from build123d import *

# Parameters (mm, degrees)
BOSS_EXTRUDE1_DEPTH         = 2.75
FILLET1_R                   = 12.7
SKETCH5_R                   = 1.3890625
CUT_EXTRUDE4_DEPTH          = 3.75
CIRPATTERN2_COUNT           = 3
CIRPATTERN2_COPY_1_SKETCH_R = 1.3890625
CIRPATTERN2_COPY_1_DEPTH    = 3.75
CIRPATTERN2_COPY_2_SKETCH_R = 1.3890625
CIRPATTERN2_COPY_2_DEPTH    = 3.75


with BuildPart() as part:
    # Sketch1 → Boss-Extrude1 (new body)
    with BuildSketch(Plane(origin=(0, 0, 0), x_dir=(1, 0, 0), z_dir=(0, 1, 0))):
        Polygon((-22.265317244, 97.17689372), (22.265317244, 97.17689372), (95.290317244, -29.306116503), (73.025, -67.870777217), (-73.025, -67.870777217), (-95.290317244, -29.306116503), align=None)
    extrude(amount=BOSS_EXTRUDE1_DEPTH)

    # Fillet1
    fillet1_edges = [part.edges().sort_by_distance(p)[0] for p in [
        (-22.265317244, 1.375, -97.17689372),
        (22.265317244, 1.375, -97.17689372),
        (95.290317244, 1.375, 29.306116503),
        (73.025, 1.375, 67.870777217),
        (-73.025, 1.375, 67.870777217),
        (-95.290317244, 1.375, 29.306116503),
    ]]
    fillet(fillet1_edges, radius=FILLET1_R)

    # Sketch5 → Cut-Extrude4 (cut, through all)
    with BuildSketch(Plane(origin=(0, 2.75, 0), x_dir=(1, 0, 0), z_dir=(0, 1, 0))):
        with Locations((21.7, -43.775677217)):
            Circle(SKETCH5_R)
        with Locations((21.7, -55.775677217)):
            Circle(SKETCH5_R)
        with Locations((39.7, -43.775677217)):
            Circle(SKETCH5_R)
        with Locations((39.7, -55.775677217)):
            Circle(SKETCH5_R)
    cut_extrude4 = extrude(amount=-CUT_EXTRUDE4_DEPTH, mode=Mode.SUBTRACT)

    # Mirror1: Cut-Extrude4 across plane
    add(cut_extrude4.mirror(Plane(origin=(0, 0, 0), x_dir=(0, 0, 1), z_dir=(1, 0, 0))), mode=Mode.SUBTRACT)

    # CirPattern2: Cut-Extrude4 ×3 about axis
    cirpattern2_axis = Axis((0, 0, 0), (0, 1, 0))
    for i in range(1, CIRPATTERN2_COUNT):
        add(cut_extrude4.rotate(cirpattern2_axis, i * 360 / CIRPATTERN2_COUNT), mode=Mode.SUBTRACT)

    # CirPattern2 copy 1 sketch → CirPattern2 copy 1 (cut, through all)
    with BuildSketch(Plane(origin=(0, 2.75, 0), x_dir=(0.5, 0, 0.866025404), z_dir=(0, 1, 0))):
        with Locations((21.7, 43.775677217)):
            Circle(CIRPATTERN2_COPY_1_SKETCH_R)
        with Locations((21.7, 55.775677217)):
            Circle(CIRPATTERN2_COPY_1_SKETCH_R)
        with Locations((39.7, 43.775677217)):
            Circle(CIRPATTERN2_COPY_1_SKETCH_R)
        with Locations((39.7, 55.775677217)):
            Circle(CIRPATTERN2_COPY_1_SKETCH_R)
    extrude(amount=-CIRPATTERN2_COPY_1_DEPTH, mode=Mode.SUBTRACT)

    # CirPattern2 copy 2 sketch → CirPattern2 copy 2 (cut, through all)
    with BuildSketch(Plane(origin=(0, 2.75, 0), x_dir=(0.5, 0, -0.866025404), z_dir=(0, 1, 0))):
        with Locations((21.7, 43.775677217)):
            Circle(CIRPATTERN2_COPY_2_SKETCH_R)
        with Locations((21.7, 55.775677217)):
            Circle(CIRPATTERN2_COPY_2_SKETCH_R)
        with Locations((39.7, 43.775677217)):
            Circle(CIRPATTERN2_COPY_2_SKETCH_R)
        with Locations((39.7, 55.775677217)):
            Circle(CIRPATTERN2_COPY_2_SKETCH_R)
    extrude(amount=-CIRPATTERN2_COPY_2_DEPTH, mode=Mode.SUBTRACT)


solid = part.part
Work out the finished part from the listing and answer in its coordinate system (mm). Coordinates: 2 decimals unless noted, no trailing zeros. Write each loop counter-clockwise with the first axis right and the second up, starting at its lowest first coordinate (ties: lowest second). Pieces come first, ordered by that corner, then holes. Notation, with made-up numbers: M 5,-12.75 L 16,-12.75 A25 cw 16,7.25 Z; hole C 86,81 d10. An arc over 180 degrees is marked long. Answer as CSV lines item,"result". Start each with the question number.
Item 1: Section B-B on z = -52 is taken. Write down the section's boundary in (x, y), and give its area (3 significant figures).
Item 2: Consider L1, parallel to Z at x = -58, y = 1.5; L2, parallel to X at y = 1.1, z = -46; L3, parallel to Z at x = -58.5, y = 0.7. Determine where each line is inside the solid, lowest interval first.
Item 3: Section A-A on y = 0.45 is taken. Give the number of separate pieces and of enclosed holes in the cut face, and give its area (3 significant figures).
Checks:
1,outline,"M -48.35,0 L 48.35,0 L 48.35,2.75 L -48.35,2.75 Z"
1,area,"266 mm²"
2,L1,"z = -35.28 to -9.87, -8.32 to 11.13, 13.86 to 67.87"
2,L2,"x = -51.81 to -38.66, -36.24 to 36.24, 38.66 to 51.81"
2,L3,"z = -34.42 to -10.32, -7.87 to 11.32, 13.67 to 67.87"
3,separate pieces,"1"
3,enclosed holes,"24"
3,area,"21,200 mm²"
